Answer from the drawing. Dimensions are ordinates in mm from the lowest x, y and z of the part. Round coordinates to 2 decimals unless told otherwise and drop trailing zeros. Write each loop counter-clockwise with the first axis right and the second up, starting at its lowest first coordinate (ties: lowest second). Pieces come first, ordered by that corner, then holes.
1. Flat-ended cylindrical pins translate along their axes: pin 1 Ø3.5 at (y, z) = (5, 11.5) entering from +X; pin 2 Ø3 at (x, z) = (7.5, 10) entering from +Y; pin 3 Ø7 at (y, z) = (6, 10) entering from -X. Find the tip coordinate at first contact, or state that the pin passes through.
2. Find section C-C (y = 6). Write down the section's boundary in (x, z) (3 decimals).
3. Find section D-D (z = 17.5). Write down the section's boundary in (x, y), and give its area (3 significant figures).
4. Find section B-B (x = 40.5). Write down the section's boundary in (y, z).
5. Find section A-A (y = 32.5). Write down the section's boundary in (x, z), and give its area (3 significant figures).
6. Straight lines are drawn through the part: probe 1 along Z at (x, y) = (56, 6); probe 2 along X at (y, z) = (57, 9.75); probe 3 along Y at (x, z) = (41, 12.5). For each, find the intervals that lie inside material, in ascending order.
7. Determine the mould class of the marked faces 1, 2, 3 and 4 for opening direction Y: pulls with the +Y half, pulls with the -Y half, needs draft (parallel to the pull), parting line crosses it, or undercut.
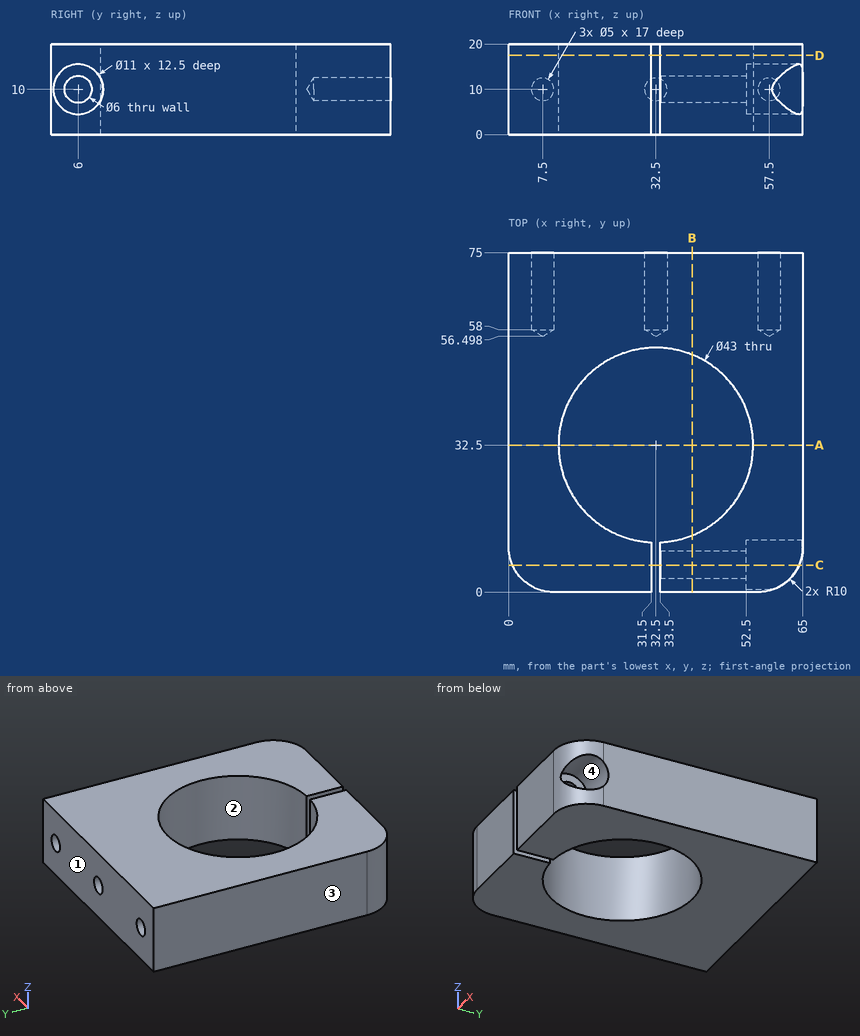
Worked answers:
1. pin 1: stops at x = 52.5
1. pin 2: stops at y = 57.4
1. pin 3: stops at x = 0.01
2. outline: (0.835, 0) - (31.5, 0) - (31.5, 20) - (0.835, 20) - close; (33.5, 0) - (64.165, 0) - (64.165, 4.5) - (52.5, 4.5) - (52.5, 7) - (33.5, 7) - close; (33.5, 13) - (52.5, 13) - (52.5, 15.5) - (64.165, 15.5) - (64.165, 20) - (33.5, 20) - close
3. outline: (0, 10) arc R10 ccw to (10, 0) - (31.5, 0) - (31.5, 11.02) arc R21.5 cw (long way) to (33.5, 11.02) - (33.5, 0) - (55, 0) arc R10 ccw to (65, 10) - (65, 75) - (0, 75) - close
3. area: 3,360 mm2
4. outline: (0, 0) - (12.54, 0) - (12.54, 20) - (0, 20) - close; (52.46, 0) - (75, 0) - (75, 20) - (52.46, 20) - close; hole circle Ø6 at (6, 10)
5. outline: (0, 0) - (11, 0) - (11, 20) - (0, 20) - close; (54, 0) - (65, 0) - (65, 20) - (54, 20) - close
5. area: 440 mm2
6. probe 1: z = 0 to 4.5, 15.5 to 20
6. probe 2: x = 0 to 6.7, 8.3 to 31.7, 33.3 to 56.7, 58.3 to 65
6. probe 3: y = 0 to 4.34, 7.66 to 12.75, 52.25 to 75
7. face 1: pulls with the +Y half
7. face 2: undercut
7. face 3: needs draft
7. face 4: undercut
